Input: part model. Units: mm. Frame: model coordinates. Face numbers are marked on the shaded views. A direction names the side the tool comes from. Give positions to 0.01 mm unless a question says otherwise; leave off trailing zeros. Loops run counter-clockwise (first coordinate to the right, second up) from the corner with the lowest first, then second, coordinate; pieces in that order, holes last. Notation, with made-up numbers: (34, 22) -> (79, 22) arc R17 cw to (79, 34) -> close; hole circle Ø1 at (12, 45). An arc over 180 degrees is marked (long way). Answer as a JSON object with one key per item and string values.
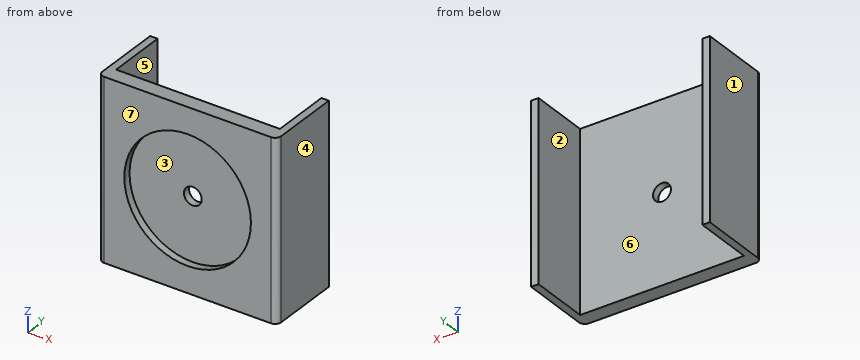
```python
from build123d import *

# Parameters (mm, degrees)
F0_W     = 152.4
F0_H     = 152.4
F1_DEPTH = 12.7
F2_R     = 53.975
F3_DEPTH = 6.35
F4_W     = 6.35
F4_H     = 50.8
F5_DEPTH = 152.4
F6_R     = 7.62
F7_DEPTH = 25.4
F8_R     = 5.08
F9_R     = 5.08


with BuildPart() as f1:
    # F0 (on Front) → F1 (new body)
    with BuildSketch(Plane.XZ):
        with Locations((-76.2, 76.2)):
            Rectangle(F0_W, F0_H)
    extrude(amount=F1_DEPTH)

    # F2 (on face) → F3 (cut)
    with BuildSketch(Plane.XZ.offset(12.7)):
        with Locations((-76.2, 76.2)):
            Circle(F2_R)
    extrude(amount=-F3_DEPTH, mode=Mode.SUBTRACT)

    # F4 (on face) → F5 (join)
    with BuildSketch(Plane(origin=(0, 0, 0), x_dir=(1, 0, 0), z_dir=(0, 0, -1))):
        with Locations((-149.225, -25.4)):
            Rectangle(F4_W, F4_H)
        with Locations((-3.175, -25.4)):
            Rectangle(F4_W, F4_H)
    extrude(amount=-F5_DEPTH)

    # F6 (on face) → F7 (cut)
    with BuildSketch(Plane.XZ.offset(6.35)):
        with Locations((-76.2, 76.2)):
            Circle(F6_R)
    extrude(amount=-F7_DEPTH, mode=Mode.SUBTRACT)

    # F8
    f8_edges = [f1.edges().sort_by_distance(p)[0] for p in [
        (-152.4, -12.7, 76.2),
    ]]
    fillet(f8_edges, radius=F8_R)

    # F9
    f9_edges = [f1.edges().sort_by_distance(p)[0] for p in [
        (0, -12.7, 76.2),
    ]]
    fillet(f9_edges, radius=F9_R)


solid = f1.part
```
Q1. Pin query (flat end, axial travel): pin 1 (10 mm diameter, centred on x = -107.5, z = 87.5, fed in from -Y). Return the tip coordinate at first contact, or that it passes through.
Evaluation:
{"pin 1": "stops at y = -6.35"}
Q2. Access query for the marked faces 1, 2 and 3. Directions: +Z, -Z, +X, -X, +Y, -Y. A direction counts if a zero-diameter tool reaches every point of the face in a straight line with its end or side. Return the directions, or none.
Evaluation:
{"face 1": "+Z, -Z, -X, +Y, -Y", "face 2": "+Z, -Z, +Y", "face 3": "-Y"}
Q3. Section A-A, the plane x = -76.2. Return the cut outline in (y, z) (3 decimals), then the cut area to 3 significant figures.
Evaluation:
{"outline": "(-12.7, 0) -> (0, 0) -> (0, 68.58) -> (-6.35, 68.58) -> (-6.35, 22.225) -> (-12.7, 22.225) -> close; (-12.7, 130.175) -> (-6.35, 130.175) -> (-6.35, 83.82) -> (0, 83.82) -> (0, 152.4) -> (-12.7, 152.4) -> close", "area": "1,150 mm2"}
Q4. Ray query, line 1 along Z through (x, y) = (-76.2, -1.25); line 2 along X through (y, z) = (19.5, 129); line 3 along Z through (x, y) = (-76, -9). Return the intervals inside material, ascending.
Evaluation:
{"line 1": "z = 0 to 68.58, 83.82 to 152.4", "line 2": "x = -152.4 to -146.05, -6.35 to 0", "line 3": "z = 0 to 22.23, 130.17 to 152.4"}
Q5. Section D-D, the plane x = -93.5. Return the cut outline in (y, z), then the cut area to 3 significant figures.
Evaluation:
{"outline": "(-12.7, 0) -> (0, 0) -> (0, 152.4) -> (-12.7, 152.4) -> (-12.7, 127.33) -> (-6.35, 127.33) -> (-6.35, 25.07) -> (-12.7, 25.07) -> close", "area": "1,290 mm2"}
Q6. Section C-C, the plane z = 38. Return the cut outline in (x, y).
Evaluation:
{"outline": "(-152.4, -7.62) arc R5.08 ccw to (-147.32, -12.7) -> (-114.33, -12.7) -> (-114.33, -6.35) -> (-38.07, -6.35) -> (-38.07, -12.7) -> (-5.08, -12.7) arc R5.08 ccw to (0, -7.62) -> (0, 50.8) -> (-6.35, 50.8) -> (-6.35, 0) -> (-146.05, 0) -> (-146.05, 50.8) -> (-152.4, 50.8) -> close"}
Q7. Section B-B, the plane z = 76.2. Return the cut outline in (x, y) (3 decimals), then the cut area to 3 significant figures.
Evaluation:
{"outline": "(-152.4, -7.62) arc R5.08 ccw to (-147.32, -12.7) -> (-130.175, -12.7) -> (-130.175, -6.35) -> (-83.82, -6.35) -> (-83.82, 0) -> (-146.05, 0) -> (-146.05, 50.8) -> (-152.4, 50.8) -> close; (-68.58, -6.35) -> (-22.225, -6.35) -> (-22.225, -12.7) -> (-5.08, -12.7) arc R5.08 ccw to (0, -7.62) -> (0, 50.8) -> (-6.35, 50.8) -> (-6.35, 0) -> (-68.58, 0) -> close", "area": "1,790 mm2"}
Q8. Draft query along X for the marked faces 4, 5, 6 and 7. Return one class per face: +X half, -X half, draft (parallel to the pull), parting line (faces both ways), or undercut.
Evaluation:
{"face 4": "+X half", "face 5": "undercut", "face 6": "undercut", "face 7": "draft"}
